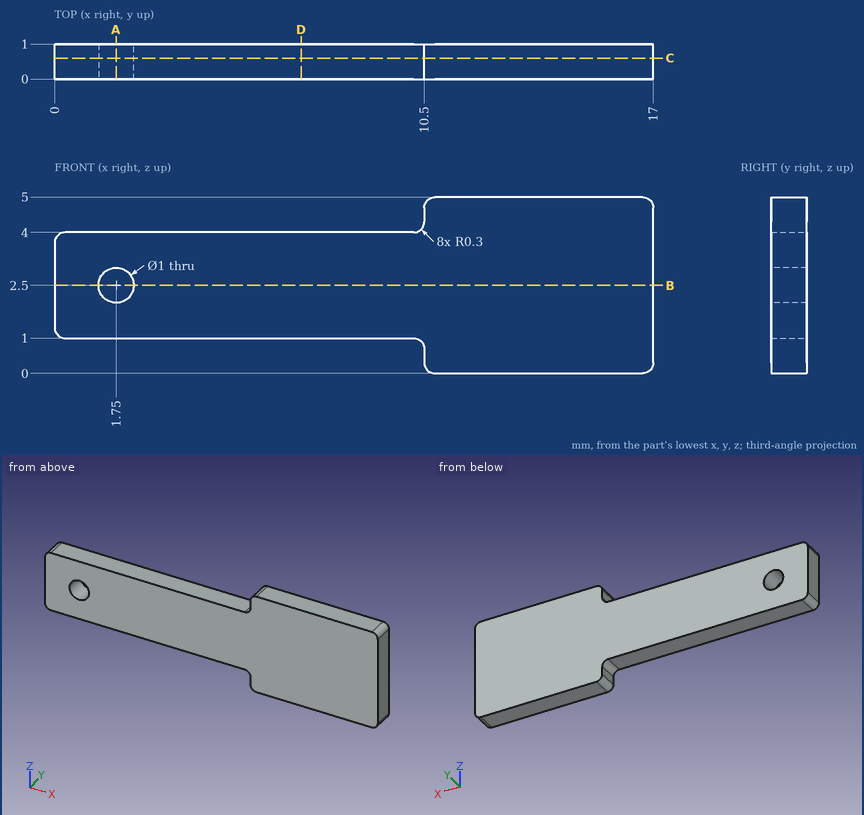
Drawing for the job (mm, zero at the part's lowest x, y, z). Round coordinates to 2 decimals unless told otherwise and drop trailing zeros. Write each loop counter-clockwise with the first axis right and the second up, starting at its lowest first coordinate (ties: lowest second). Pieces come first, ordered by that corner, then holes. Notation, with made-up numbers: (51, 5) - (63, 5) arc R14 ccw to (63, 31) - close; hole circle Ø8 at (60, 38). An arc over 180 degrees is marked (long way). Write item = value, one per line. Start each with the question number.
Q1. Band-saw the part on C-C (y = 0.6). Give the cut face in (x, z).
Q2. Band-saw the part on A-A (x = 1.75). Give the cut face in (y, z).
Q3. Band-saw the part on D-D (x = 7). Give the cut face in (y, z).
Q4. Drop a flat-ended pin along its axis: pin 1 (2 mm diameter, centred on x = 13.5, z = 2.5, fed in from -Y). Give the stop position or say it passes through.
Q5. Band-saw the part on B-B (z = 2.5). Give the cut face in (x, y), then the cut area to 3 significant figures.
Q6. Probe L1, parallel to X at y = 0.4, z = 2.5; L2, parallel to Z at x = 1.75, y = 0.6; L3, parallel to X at y = 0.8, z = 0.9. List the from-to ranges inside material, lowest first. Write a range as from..to.
Answers below:
q1.outline = (0, 1.3) arc R0.3 ccw to (0.3, 1) - (10.2, 1) arc R0.3 cw to (10.5, 0.7) - (10.5, 0.3) arc R0.3 ccw to (10.8, 0) - (16.7, 0) arc R0.3 ccw to (17, 0.3) - (17, 4.7) arc R0.3 ccw to (16.7, 5) - (10.8, 5) arc R0.3 ccw to (10.5, 4.7) - (10.5, 4.3) arc R0.3 cw to (10.2, 4) - (0.3, 4) arc R0.3 ccw to (0, 3.7) - close; hole circle Ø1 at (1.75, 2.5)
q2.outline = (0, 1) - (1, 1) - (1, 2) - (0, 2) - close; (0, 3) - (1, 3) - (1, 4) - (0, 4) - close
q3.outline = (0, 1) - (1, 1) - (1, 4) - (0, 4) - close
q4.pin_1 = 0
q5.outline = (0, 0) - (1.25, 0) - (1.25, 1) - (0, 1) - close; (2.25, 0) - (17, 0) - (17, 1) - (2.25, 1) - close
q5.area = 16.0 mm2
q6.L1 = 0..1.25, 2.25..17
q6.L2 = 1..2, 3..4
q6.L3 = 10.42..17
